```python
from build123d import *

# Parameters (mm, degrees)
PAD_DEPTH       = 14.5
POCKET_DEPTH    = 5
CHAMFER_SIZE    = 3
CHAMFER001_SIZE = 3


with BuildPart() as part:
    # Sketch → Pad (new body)
    with BuildSketch(Plane.XZ):
        with BuildLine():
            ThreePointArc((-3.316625, 10), (-5.840963, 6.372281), (-5.196152, 2))
            Line((-5.196152, 2), (-5.196152, 0))
            Line((-13.196152, 0), (-5.196152, 0))
            Line((-13.196152, 2), (-13.196152, 0))
            Line((-7.196152, 2), (-13.196152, 2))
            Line((-7.196152, 11.5), (-7.196152, 2))
            Line((7.196152, 11.5), (-7.196152, 11.5))
            Line((7.196152, 2), (7.196152, 11.5))
            Line((13.196152, 2), (7.196152, 2))
            Line((13.196152, 0), (13.196152, 2))
            Line((5.196152, 0), (13.196152, 0))
            Line((5.196152, 2), (5.196152, 0))
            ThreePointArc((5.196152, 2), (5.840963, 6.372281), (3.316625, 10))
            Line((-3.316625, 10), (3.316625, 10))
        make_face()
    extrude(amount=PAD_DEPTH)

    # Sketch001 (on Face7 of Pad) → Pocket (cut)
    with BuildSketch(Plane(origin=(0, 0, 2), x_dir=(-1, 0, 0), z_dir=(0, 0, 1))):
        with BuildLine():
            ThreePointArc((-11.095237, 8.300175), (-10, 5.3), (-8.904763, 8.300175))
            Line((-10, 9.222777), (-8.904763, 8.300175))
            Line((-11.095237, 8.300175), (-10, 9.222777))
        make_face()
    pocket = extrude(amount=-POCKET_DEPTH, mode=Mode.SUBTRACT)

    # Mirrored: Pocket across YZ
    add(pocket.mirror(Plane.YZ), mode=Mode.SUBTRACT)

    # Chamfer
    chamfer_edges = [part.edges().sort_by_distance(p)[0] for p in [
        (-7.196152, -7.25, 11.5),
        (7.196152, -7.25, 11.5),
    ]]
    chamfer(chamfer_edges, length=CHAMFER_SIZE)

    # Chamfer001
    chamfer001_edges = [part.edges().sort_by_distance(p)[0] for p in [
        (-13.196152, -14.5, 1),
        (13.196152, -14.5, 1),
        (13.196152, 0, 1),
        (-13.196152, 0, 1),
    ]]
    chamfer(chamfer001_edges, length=CHAMFER001_SIZE)


solid = part.part
```
Input: part model. Units: mm. Frame: model coordinates. A direction names the side the tool comes from. Coordinates: 2 decimals unless noted, no trailing zeros. Write each loop counter-clockwise with the first axis right and the second up, starting at its lowest first coordinate (ties: lowest second). Pieces come first, ordered by that corner, then holes. Notation, with made-up numbers: (23, 9) -> (39, 9) arc R23 cw to (39, 45) -> close; hole circle Ø2 at (15, 34.25). An arc over 180 degrees is marked (long way). Write each question's results on one line, items separated by ' | '.
Item 1: Section query C-C on z = 7.5. Return loops of the section in (x, y).
Conclusion:
outline: (-7.2, -14.5) -> (-5.45, -14.5) -> (-5.45, 0) -> (-7.2, 0) -> close; (5.45, -14.5) -> (7.2, -14.5) -> (7.2, 0) -> (5.45, 0) -> close
Item 2: Pin query (flat end, axial travel): pin 1 Ø2 at (x, y) = (-2.5, -5.5) entering from -Z; pin 2 Ø3 at (x, y) = (-11.5, -9.5) entering from +Z; pin 3 Ø2 at (x, y) = (10, -7) entering from +Z; pin 4 Ø1 at (x, y) = (-3.5, -3) entering from -Z. Return the tip coordinate at first contact, or that it passes through.
Conclusion:
pin 1: stops at z = 9.87 | pin 2: stops at z = 2 | pin 3: passes through | pin 4: stops at z = 9.47
Item 3: Material intervals for probe 1 along X at (y, z) = (-7, 1.45); probe 2 along X at (y, z) = (-10.25, 0.75); probe 3 along Z at (x, y) = (10, -13.25), sorted ascending.
Conclusion:
probe 1: x = -13.2 to -11.7, -8.3 to -5.2, 5.2 to 8.3, 11.7 to 13.2 | probe 2: x = -13.2 to -5.2, 5.2 to 13.2 | probe 3: z = 0 to 2
Item 4: Mould query, pull axis Z, two halves, no side actions, for faces 6 (the cylindrical face through (-5.826, -7.148, 6.434)), 7 (the flat face through (-5.675, -7.148, 10.021)), 8 (the flat face through (13.196, -7, 1)). Classes: +Z half, -Z half, draft (parallel to the pull), parting line (faces both ways), or undercut.
Conclusion:
face 6: undercut | face 7: +Z half | face 8: draft
Item 5: Set-up query: faces 1 (the flat face through (9.5, -8.8, 1)), 2 (the flat face through (-7.196, -7, 5)), 3 (the flat face through (7.196, -7, 5)), 4 (the flat face through (11.675, -13.021, 0.986)), 5 (the flat face through (5.196, -7, 1)). Return all of +Z, -Z, +X, -X, +Y, -Y with unobstructed straight access to the full face (end or side cutting, diameter ignored); none if empty.
Conclusion:
face 1: +Z, -Z | face 2: +Z, -X, +Y, -Y | face 3: +Z, +X, +Y, -Y | face 4: +Z, -Z, +X, -Y | face 5: -Z, +Y, -Y
Item 6: Section query B-B on x = -10.5. Return loops of the section in (y, z), plus the area to 3 significant figures.
Conclusion:
outline: (-14.2, 0) -> (-8.8, 0) -> (-8.8, 2) -> (-14.2, 2) -> close; (-5.38, 0) -> (-0.3, 0) -> (-0.3, 2) -> (-5.38, 2) -> close | area: 20.9 mm^2
Item 7: Section query D-D on y = -1.75. Return loops of the section in (x, z).
Conclusion:
outline: (-11.95, 0) -> (-5.2, 0) -> (-5.2, 2) arc R6 cw to (-3.32, 10) -> (3.32, 10) arc R6 cw to (5.2, 2) -> (5.2, 0) -> (11.95, 0) -> (11.95, 2) -> (7.2, 2) -> (7.2, 8.5) -> (4.2, 11.5) -> (-4.2, 11.5) -> (-7.2, 8.5) -> (-7.2, 2) -> (-11.95, 2) -> close
Item 8: Section query A-A on y = -7. Return loops of the section in (x, z), plus the area to 3 significant figures.
Conclusion:
outline: (-13.2, 0) -> (-11.7, 0) -> (-11.7, 2) -> (-13.2, 2) -> close; (-8.3, 0) -> (-5.2, 0) -> (-5.2, 2) arc R6 cw to (-3.32, 10) -> (3.32, 10) arc R6 cw to (5.2, 2) -> (5.2, 0) -> (8.3, 0) -> (8.3, 2) -> (7.2, 2) -> (7.2, 8.5) -> (4.2, 11.5) -> (-4.2, 11.5) -> (-7.2, 8.5) -> (-7.2, 2) -> (-8.3, 2) -> close; (11.7, 0) -> (13.2, 0) -> (13.2, 2) -> (11.7, 2) -> close | area: 59.6 mm^2
